Geometry: final body of the model. Coordinates: model frame, mm. Face numbers are marked on the shaded views. A direction names the side the tool comes from. Give positions to 0.01 mm unless a question says otherwise; leave off trailing zeros. Write each loop counter-clockwise with the first axis right and the second up, starting at its lowest first coordinate (ties: lowest second). Pieces come first, ordered by that corner, then holes. Notation, with made-up numbers: (-21, 37.5) -> (24, 37.5) arc R16 ccw to (24, 57.5) -> close; hole circle Ø3 at (23, 31.5). An arc over 180 degrees is marked (long way). Answer as a JSON object with one key per item and string values.
from build123d import *

# Parameters (mm, degrees)
BOSS_EXTRUDE7_DEPTH = 10
SKETCH1_23_R        = 65.000000017
SKETCH1_23_R_2      = 4.125
BOSS_EXTRUDE8_DEPTH = 10
CUT_EXTRUDE1_START  = 65
SKETCH16_R          = 2.5
CUT_EXTRUDE1_DEPTH  = 20
BOSS_EXTRUDE9_START = -0.5
SKETCH17_R          = 12.5
SKETCH17_R_2        = 3.175
BOSS_EXTRUDE9_DEPTH = 5.5
FILLET1_R           = 5
SKETCH18_R          = 2.5
SKETCH18_R_2        = 3.5
CUT_EXTRUDE2_DEPTH  = 10
SKETCH20_R          = 2.625
CUT_EXTRUDE11_DEPTH = 25


with BuildPart() as part:
    # Sketch1 → Boss-Extrude7 (new body)
    with BuildSketch(Plane(origin=(0, 0, 0), x_dir=(1, 0, 0), z_dir=(0, 1, 0))):
        with BuildLine():
            ThreePointArc((-10.099280768, -64.210626285), (-56.291651246, -32.5), (-60.65767394, 23.359079438))
            Line((-60.65767394, 23.359079438), (-64.257390064, 17.124188218))
            ThreePointArc((-64.257390064, 17.124188218), (-57.590689352, -33.25), (-17.298713017, -64.210626285))
            Line((-17.298713017, -64.210626285), (-10.099280768, -64.210626285))
        make_face()
        with BuildLine():
            Line((-64.257390064, 17.124188218), (-60.65767394, 23.359079438))
            ThreePointArc((-60.65767394, 23.359079438), (-60.639599413, 23.405960416), (-60.621488653, 23.452827409))
            Line((-60.621488653, 23.452827409), (-61.93581913, 24.211656463))
            ThreePointArc((-61.93581913, 24.211656463), (-63.196040724, 20.700493636), (-64.257390064, 17.124188218))
        make_face()
        with BuildLine():
            ThreePointArc((-60.621488653, 23.452827409), (-59.667920988, 25.782536821), (-58.624860802, 28.073576473))
            ThreePointArc((-58.624860802, 28.073576473), (-54.991019149, 34.65527107), (-50.621488653, 40.773335485))
            Line((-50.621488653, 40.773335485), (-51.93581913, 41.532164539))
            ThreePointArc((-51.93581913, 41.532164539), (-57.590689352, 33.25), (-61.93581913, 24.211656463))
            Line((-61.93581913, 24.211656463), (-60.621488653, 23.452827409))
        make_face()
        with BuildLine():
            ThreePointArc((-50.621488653, 40.773335485), (-50.589956027, 40.812453359), (-50.558393172, 40.851546848))
            Line((-50.558393172, 40.851546848), (-46.958677048, 47.086438068))
            ThreePointArc((-46.958677048, 47.086438068), (-49.525173722, 44.379129868), (-51.93581913, 41.532164539))
            Line((-51.93581913, 41.532164539), (-50.621488653, 40.773335485))
        make_face()
        with BuildLine():
            Line((-46.958677048, 47.086438068), (-50.558393172, 40.851546848))
            ThreePointArc((-50.558393172, 40.851546848), (0, 65), (50.558393172, 40.851546848))
            Line((50.558393172, 40.851546848), (46.958677048, 47.086438068))
            ThreePointArc((46.958677048, 47.086438068), (0, 66.5), (-46.958677048, 47.086438068))
        make_face()
        with BuildLine():
            Line((46.958677048, 47.086438068), (50.558393172, 40.851546848))
            ThreePointArc((50.558393172, 40.851546848), (50.589956027, 40.812453359), (50.621488653, 40.773335485))
            Line((50.621488653, 40.773335485), (51.93581913, 41.532164539))
            ThreePointArc((51.93581913, 41.532164539), (49.525173722, 44.379129868), (46.958677048, 47.086438068))
        make_face()
        with BuildLine():
            Line((51.93581913, 41.532164539), (50.621488653, 40.773335485))
            ThreePointArc((50.621488653, 40.773335485), (52.162292355, 38.782666956), (53.624860802, 36.733830511))
            ThreePointArc((53.624860802, 36.733830511), (57.507854696, 30.295984028), (60.621488653, 23.452827409))
            Line((60.621488653, 23.452827409), (61.93581913, 24.211656463))
            ThreePointArc((61.93581913, 24.211656463), (57.590689352, 33.25), (51.93581913, 41.532164539))
        make_face()
        with BuildLine():
            ThreePointArc((64.257390064, 17.124188218), (63.196040724, 20.700493636), (61.93581913, 24.211656463))
            Line((61.93581913, 24.211656463), (60.621488653, 23.452827409))
            ThreePointArc((60.621488653, 23.452827409), (60.639599413, 23.405960416), (60.65767394, 23.359079438))
            Line((60.65767394, 23.359079438), (64.257390064, 17.124188218))
        make_face()
        with BuildLine():
            ThreePointArc((66.5, 0), (65.936963986, 8.635205867), (64.257390064, 17.124188218))
            Line((64.257390064, 17.124188218), (60.65767394, 23.359079438))
            ThreePointArc((60.65767394, 23.359079438), (63.90519856, 11.879629495), (65, 0))
            ThreePointArc((65, 0), (49.40371064, -42.240660211), (10.099280768, -64.210626285))
            Line((10.099280768, -64.210626285), (17.298713017, -64.210626285))
            ThreePointArc((17.298713017, -64.210626285), (52.785482927, -40.44678964), (66.5, 0))
        make_face()
        with BuildLine():
            ThreePointArc((-10, -64.226162893), (-10.049643386, -64.218413775), (-10.099280768, -64.210626285))
            Line((-10.099280768, -64.210626285), (-17.298713017, -64.210626285))
            ThreePointArc((-17.298713017, -64.210626285), (-13.670867002, -65.079623504), (-10, -65.743821002))
            Line((-10, -65.743821002), (-10, -64.226162893))
        make_face()
        with BuildLine():
            ThreePointArc((5, -64.807406984), (-2.516835548, -64.951255098), (-10, -64.226162893))
            Line((-10, -64.226162893), (-10, -65.743821002))
            ThreePointArc((-10, -65.743821002), (0, -66.5), (10, -65.743821002))
            Line((10, -65.743821002), (10, -64.226162893))
            ThreePointArc((10, -64.226162893), (7.505628633, -64.565203777), (5, -64.807406984))
        make_face()
        with BuildLine():
            Line((10, -64.226162893), (10, -65.743821002))
            ThreePointArc((10, -65.743821002), (13.670867002, -65.079623504), (17.298713017, -64.210626285))
            Line((17.298713017, -64.210626285), (10.099280768, -64.210626285))
            ThreePointArc((10.099280768, -64.210626285), (10.049643386, -64.218413775), (10, -64.226162893))
        make_face()
    extrude(amount=BOSS_EXTRUDE7_DEPTH)

    # Sketch1<23> → Boss-Extrude8 (add)
    with BuildSketch(Plane(origin=(0, 0, 0), x_dir=(1, 0, 0), z_dir=(0, 1, 0))):
        with Locations((-3e-09, 1.7e-08)):
            Circle(SKETCH1_23_R)
        with Locations(Location((0, 0, 0), (0, 0, 270))):
            Circle(SKETCH1_23_R_2, mode=Mode.SUBTRACT)
    extrude(amount=BOSS_EXTRUDE8_DEPTH)

    # Sketch16 → Cut-Extrude1 (cut)
    with BuildSketch(Plane.XZ.offset(-75).offset(CUT_EXTRUDE1_START)):
        with Locations(Location((36.217182386, -20.91, 0), (0, 0, 90))):
            Circle(SKETCH16_R)
        with Locations(Location((49.796460718, -28.75, 0), (0, 0, 90))):
            Circle(SKETCH16_R)
        with Locations(Location((-40.967182386, -12.682758664, 0), (0, 0, 90))):
            Circle(SKETCH16_R)
        with Locations(Location((-36.217182386, -20.91, 0), (0, 0, 90))):
            Circle(SKETCH16_R)
        with Locations(Location((-49.796460718, -28.75, 0), (0, 0, 90))):
            Circle(SKETCH16_R)
        with Locations(Location((0, 41.82, 0), (0, 0, 90))):
            Circle(SKETCH16_R)
        with Locations(Location((0, 57.5, 0), (0, 0, 90))):
            Circle(SKETCH16_R)
        with Locations(Location((-31.467182386, -29.137241336, 0), (0, 0, 90))):
            Circle(SKETCH16_R)
        with Locations(Location((-45.046460718, -36.977241336, 0), (0, 0, 90))):
            Circle(SKETCH16_R)
        with Locations(Location((-54.546460718, -20.522758664, 0), (0, 0, 90))):
            Circle(SKETCH16_R)
        with Locations(Location((9.5, 41.82, 0), (0, 0, 90))):
            Circle(SKETCH16_R)
        with Locations(Location((-9.5, 41.82, 0), (0, 0, 90))):
            Circle(SKETCH16_R)
        with Locations(Location((-9.5, 57.5, 0), (0, 0, 90))):
            Circle(SKETCH16_R)
        with Locations(Location((9.5, 57.5, 0), (0, 0, 90))):
            Circle(SKETCH16_R)
        with Locations(Location((31.467182386, -29.137241336, 0), (0, 0, 90))):
            Circle(SKETCH16_R)
        with Locations(Location((40.967182386, -12.682758664, 0), (0, 0, 90))):
            Circle(SKETCH16_R)
        with Locations(Location((54.546460718, -20.522758664, 0), (0, 0, 90))):
            Circle(SKETCH16_R)
        with Locations(Location((45.046460718, -36.977241336, 0), (0, 0, 90))):
            Circle(SKETCH16_R)
    extrude(amount=CUT_EXTRUDE1_DEPTH, mode=Mode.SUBTRACT)

    # Sketch17 → Boss-Extrude9 (add)
    with BuildSketch(Plane(origin=(0, 10, 0), x_dir=(1, 0, 0), z_dir=(0, 1, 0)).offset(BOSS_EXTRUDE9_START)):
        with Locations(Location((0, 0, 0), (0, 0, 270))):
            Circle(SKETCH17_R)
        with Locations(Location((0, 0, 0), (0, 0, 270))):
            Circle(SKETCH17_R_2, mode=Mode.SUBTRACT)
    extrude(amount=BOSS_EXTRUDE9_DEPTH)

    # Fillet1
    fillet1_edges = [part.edges().sort_by_distance(p)[0] for p in [
        (0, 10, -12.5),
    ]]
    fillet(fillet1_edges, radius=FILLET1_R - 0.0001)  # a hair under: the kernel refuses the full size

    # Sketch18 → Cut-Extrude2 (cut)
    with BuildSketch(Plane(origin=(0, 10, 0), x_dir=(1, 0, 0), z_dir=(0, 1, 0))):
        with Locations(Location((0, 56.5, 0), (0, 0, 270))):
            Circle(SKETCH18_R)
        with Locations(Location((0, 46.5, 0), (0, 0, 270))):
            Circle(SKETCH18_R)
        with Locations(Location((40.270181276, -23.25, 0), (0, 0, 270))):
            Circle(SKETCH18_R)
        with Locations(Location((48.930435314, -28.25, 0), (0, 0, 270))):
            Circle(SKETCH18_R)
        with Locations(Location((-40.270181276, -23.25, 0), (0, 0, 270))):
            Circle(SKETCH18_R)
        with Locations(Location((-48.930435314, -28.25, 0), (0, 0, 270))):
            Circle(SKETCH18_R)
        with Locations(Location((-26.035163591, -15.031408708, 0), (0, 0, 270))):
            Circle(SKETCH18_R_2)
        with Locations(Location((0, 30.062817415, 0), (0, 0, 270))):
            Circle(SKETCH18_R_2)
    extrude(amount=-CUT_EXTRUDE2_DEPTH, mode=Mode.SUBTRACT)

    # Sketch20 → Cut-Extrude11 (cut)
    with BuildSketch(Plane(origin=(0, 10, 0), x_dir=(1, 0, 0), z_dir=(0, 1, 0))):
        with Locations(Location((-20.784609691, 12, 0), (0, 0, 270))):
            Circle(SKETCH20_R)
        with Locations(Location((0, -24, 0), (0, 0, 270))):
            Circle(SKETCH20_R)
        with Locations(Location((20.784609691, 12, 0), (0, 0, 270))):
            Circle(SKETCH20_R)
    extrude(amount=-CUT_EXTRUDE11_DEPTH, mode=Mode.SUBTRACT)


solid = part.part
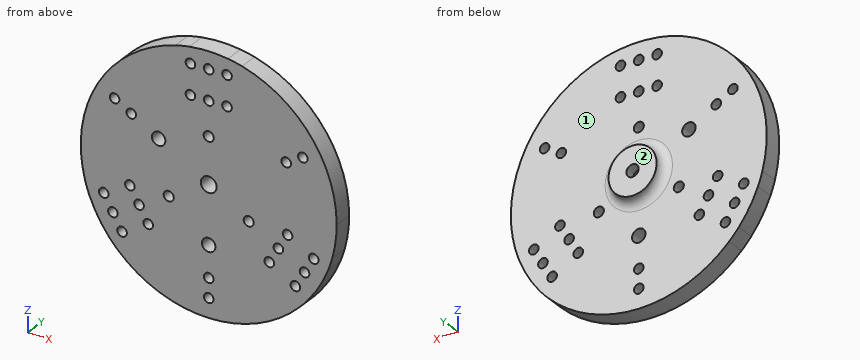
Q1. Cut plane D-D (z = -56.5). Return the cut outline in (x, y).
Values:
{"outline": "(-35.07, 0) -> (-2.5, 0) -> (-2.5, 10) -> (-35.07, 10) -> close; (2.5, 0) -> (35.07, 0) -> (35.07, 10) -> (2.5, 10) -> close"}
Q2. Material intervals for L1, parallel to X at y = 2.75, z = 0.5; L2, parallel to X at y = 9, z = 28.5; L3, parallel to Y at x = -58, z = -23, sorted ascending. Write a range as from..to.
Values:
{"L1": "-66.5..-4.09, 4.09..66.5", "L2": "-60.08..-51.42, -46.44..46.44, 51.42..60.08", "L3": "0..10"}
Q3. Cut plane A-A (z = 28.25). Return the cut outline in (x, y), and give its area (3 significant figures).
Values:
{"outline": "(-60.2, 0) -> (-51.43, 0) -> (-51.43, 10) -> (-60.2, 10) -> close; (-46.43, 0) -> (46.43, 0) -> (46.43, 10) -> (-46.43, 10) -> close; (51.43, 0) -> (60.2, 0) -> (60.2, 10) -> (51.43, 10) -> close", "area": "1,100 mm²"}
Q4. Set-up query: the marked faces 1 and 2. Return all of +Z, -Z, +X, -X, +Y, -Y with unobstructed straight access to the full face (end or side cutting, diameter ignored); none if empty.
Values:
{"face 1": "+Y", "face 2": "+Z, -Z, +X, -X, +Y"}
Q5. Cut plane B-B (z = 41.82). Return the cut outline in (x, y), and give its area (3 significant figures).
Values:
{"outline": "(-51.7, 0) -> (-12, 0) -> (-12, 10) -> (-51.7, 10) -> close; (-7, 0) -> (-2.5, 0) -> (-2.5, 10) -> (-7, 10) -> close; (2.5, 0) -> (7, 0) -> (7, 10) -> (2.5, 10) -> close; (12, 0) -> (51.7, 0) -> (51.7, 10) -> (12, 10) -> close", "area": "884 mm²"}
Q6. First-contact query: P1, Ø6, axis at x = 8, y = 9, coming from the -Z side; P2, Ø6, axis at y = 7, z = 36, coming from the -X side; P3, Ø4, axis at x = 25, z = 37.5, coming from the +Y side; P4, Ø3, axis at x = -45.05, z = -36.98, coming from the -Y side. Flat tips, straight axial feed; report the tip coordinate or a pass-through.
Values:
{"P1": "z = -66.31", "P2": "x = -57.73", "P3": "y = 10", "P4": "through"}
Q7. Cut plane C-C (x = 0). State how many separate pieces and enclosed holes the cut face has, and give its area (3 significant figures).
Values:
{"separate pieces": "8", "enclosed holes": "0", "area": "1,030 mm²"}
